from build123d import *

# Parameters (mm, degrees)
TD_SKETCH_R                             = 0.79248
TL_FEATURE_DEPTH                        = 21.0312
TDF_STD_SKETCH_W                        = 2.09296
TDF_STD_SKETCH_H                        = 2.09296
TDF_STD_FEATURE_DEPTH                   = 22.061040395
ISA_20_STD_FEATURE_DEPTH                = 22.061040395
ISA_20_STD_FEATURE_DEPTH_BACK           = 22.061040395
F_10BA_STD_FEATURE_DEPTH                = 22.061040395
F_10BA_STD_FEATURE_DEPTH_BACK           = 22.061040395
FRO_STD_FEATURE_DEPTH                   = 22.061040395
FRO_STD_FEATURE_DEPTH_BACK              = 22.061040395
C_STD_FEATURE_DEPTH                     = 22.061040395
C_STD_FEATURE_DEPTH_BACK                = 22.061040395
ERW_STD_FEATURE_DEPTH                   = 0.0254
H_STD_FEATURE_REACH                     = 22.907
H_STD_SKETCH_R                          = 0.0254
H_STD_SKETCH_3_R                        = 0.0254
FUNNEL_FINAL_DIAMETRE_STD_FEATURE_DEPTH = 2.499995
FUNNEL_FINAL_DIAMETRE_STD_FEATURE_DRAFT = -22.5
ROUND_BR_STD_FEATURE_START              = -1
ROUND_BR_STD_FEATURE_DEPTH              = 0.984425518


with BuildPart() as part:
    # TD_sketch → TL_feature (new body)
    with BuildSketch(Plane(origin=(0, 0, 0), x_dir=(1, 0, 0), z_dir=(0, 1, 0))):
        with Locations(Location((0, 0, 0), (0, 0, 270))):
            Circle(TD_SKETCH_R)
    extrude(amount=TL_FEATURE_DEPTH)

    # TDF_STD_sketch → TDF_STD_feature (cut, through all)
    with BuildSketch(Plane(origin=(0, 0, 0), x_dir=(1, 0, 0), z_dir=(0, 1, 0))):
        with Locations((-1.4224, 0)):
            Rectangle(TDF_STD_SKETCH_W, TDF_STD_SKETCH_H)
    extrude(amount=TDF_STD_FEATURE_DEPTH, mode=Mode.SUBTRACT)

    # ISA_20_STD_sketch → ISA_20_STD_feature (cut, two sides: drawn at the far end of the back side and taken through both)
    with BuildSketch(Plane(origin=(0, 0, 0), x_dir=(0, 0, -1), z_dir=(1, 0, 0)).offset(-ISA_20_STD_FEATURE_DEPTH_BACK)):
        Polygon((-12.968809457, 73.261672178), (-3.759167997, 21.0312), (-0.0508, 0), (0.0508, 0), (3.759167997, 21.0312), (12.968809457, 73.261672178), (12.968809457, -32.810750623), (-12.968809457, -32.810750623), align=None)
    extrude(amount=ISA_20_STD_FEATURE_DEPTH + ISA_20_STD_FEATURE_DEPTH_BACK, mode=Mode.SUBTRACT)

    # 10BA_STD_sketch → 10BA_STD_feature (cut, two sides: drawn at the far end of the back side and taken through both)
    with BuildSketch(Plane.XY.offset(-F_10BA_STD_FEATURE_DEPTH_BACK)):
        Polygon((-53.226091717, 0), (-0.37592, 0), (-0.24892, 0), (0.011534356, 0.036604473), (3.713447997, 21.0312), (12.890784005, 73.078458855), (91.272293615, 2.163710365), (25.155417893, -70.914748491), align=None)
    extrude(amount=F_10BA_STD_FEATURE_DEPTH + F_10BA_STD_FEATURE_DEPTH_BACK, mode=Mode.SUBTRACT)

    # FRO_STD_sketch → FRO_STD_feature (cut, two sides: drawn at the far end of the back side and taken through both)
    with BuildSketch(Plane.XY.offset(-FRO_STD_FEATURE_DEPTH_BACK)):
        with BuildLine():
            Line((-0.37592, 52.149873762), (-0.37592, 0.0254))
            ThreePointArc((-0.37592, 0.0254), (-0.368480512, 0.007439488), (-0.35052, 0))
            Line((-0.35052, 0), (51.773953762, 0))
            Line((51.773953762, 0), (-21.941183964, -73.715137726))
            Line((-21.941183964, -73.715137726), (-74.091057726, -21.565263964))
            Line((-74.091057726, -21.565263964), (-0.37592, 52.149873762))
        make_face()
    extrude(amount=FRO_STD_FEATURE_DEPTH + FRO_STD_FEATURE_DEPTH_BACK, mode=Mode.SUBTRACT)

    # C_STD_sketch → C_STD_feature (cut, two sides: drawn at the far end of the back side and taken through both)
    with BuildSketch(Plane(origin=(0, 0, 0), x_dir=(0, 0, -1), z_dir=(1, 0, 0)).offset(-C_STD_FEATURE_DEPTH_BACK)):
        with BuildLine():
            Line((-51.498419713, -8.177529753), (-0.048243287, 0))
            ThreePointArc((-0.048243287, 0), (0, 0.00381), (0.048243287, 0))
            Line((0.048243287, 0), (51.498419713, -8.177529753))
            Line((51.498419713, -8.177529753), (51.498419713, -112.369518834))
            Line((51.498419713, -112.369518834), (-51.498419713, -112.369518834))
            Line((-51.498419713, -112.369518834), (-51.498419713, -8.177529753))
        make_face()
    extrude(amount=C_STD_FEATURE_DEPTH + C_STD_FEATURE_DEPTH_BACK, mode=Mode.SUBTRACT)


with BuildPart() as body_2:
    # ERW_STD_sketch → ERW_STD_feature (new, symmetric)
    with BuildSketch(Plane.XY):
        Polygon((-0.127, 0.0762), (-0.127, 0), (-0.29718, 0), (-0.239759181, 0.0762), align=None)
    extrude(amount=ERW_STD_FEATURE_DEPTH, both=True)

    # H_STD_sketch → H_STD_feature (add, up to next)
    with BuildSketch(Plane(origin=(0.008335492, 0.154335983, 0), x_dir=(0, 0, -1), z_dir=(0.8660254037844415, 0.4999999999999953, 0)), mode=Mode.PRIVATE) as h_std_feature_sk1:
        with Locations(Location((0, 0, 0), (0, 0, 90))):
            Circle(H_STD_SKETCH_R)
    h_std_feature_tool1 = extrude(h_std_feature_sk1.sketch, amount=-H_STD_FEATURE_REACH, mode=Mode.PRIVATE) - body_2.part
    add(h_std_feature_tool1.solids().sort_by_distance((0.008335, 0.154336, 0))[0])


with BuildPart() as funnel_final_diametre_std_feature_tool:
    # H_STD_sketch<3> → funnel_final_diametre_STD_feature (with draft: the straight prism first)
    with BuildSketch(Plane(origin=(0.008335492, 0.154335983, 0), x_dir=(0, 0, -1), z_dir=(0.8660254037844415, 0.4999999999999953, 0))):
        with Locations(Location((0, 0, 0), (0, 0, 90))):
            Circle(H_STD_SKETCH_3_R)
    extrude(amount=FUNNEL_FINAL_DIAMETRE_STD_FEATURE_DEPTH)
    # funnel_final_diametre_STD_feature: the draft: its side faces are tilted about the plane it starts from
    funnel_final_diametre_std_feature_sides = [funnel_final_diametre_std_feature_tool.faces().sort_by_distance(p)[0] for p in [
        (1.103565082, 0.757337687, 0),
    ]]
    draft(funnel_final_diametre_std_feature_sides, Plane(origin=(0.008335492, 0.154335983, 0), x_dir=(0, 0, -1), z_dir=(0.8660254037844415, 0.4999999999999953, 0)), FUNNEL_FINAL_DIAMETRE_STD_FEATURE_DRAFT)


with BuildPart() as body_2_1:
    add(body_2.part)

    # funnel_final_diametre_STD_feature: add funnel_final_diametre_std_feature_tool
    add(funnel_final_diametre_std_feature_tool.part)

    # ROUND_BR_STD_feature: read off the stored shape, not the designer's step
    # ROUND_BR_STD_feature outline → ROUND_BR_STD_feature (cut)
    with BuildSketch(Plane(origin=(0, 0, 0), x_dir=(0.79863551004729, -0.601815023152052, 0), z_dir=(0.601815023152052, 0.79863551004729, 0)).offset(ROUND_BR_STD_FEATURE_START)):
        with BuildLine():
            Line((-0.237338501, -0.0254), (-0.211938501, -0.0254))
            ThreePointArc((-0.211938501, -0.0254), (-0.229899013, -0.017960512), (-0.237338501, 0))
            Line((-0.237338501, 0), (-0.237338501, -0.0254))
        make_face()
        with BuildLine():
            Line((-0.237338501, 0.0254), (-0.237338501, 0))
            ThreePointArc((-0.237338501, 0), (-0.229899013, 0.017960512), (-0.211938501, 0.0254))
            Line((-0.211938501, 0.0254), (-0.237338501, 0.0254))
        make_face()
    extrude(amount=ROUND_BR_STD_FEATURE_DEPTH, mode=Mode.SUBTRACT)


with BuildPart() as part_1:
    add(part.part)

    # COMBINE_STD_feature: cut body 2
    add(body_2_1.part, mode=Mode.SUBTRACT)


solid = part_1.part
Here's how the part is built. I have some questions about the finished solid (model axes, mm). Coordinates: 2 decimals unless noted, no trailing zeros. Loops run counter-clockwise (first coordinate to the right, second up) from the corner with the lowest first, then second, coordinate; pieces in that order, holes last. Notation, with made-up numbers: (-5.5, -1) -> (37.5, -1) arc R30 ccw to (37.5, 22) -> close; hole circle Ø6 at (34, 1.5). An arc over 180 degrees is marked (long way). Use one line per item in the form item = value. Start each with the question number.
(1) If we section it at C-C (y = 1.75): Please give me the cut outline in (x, z).
(2) If we section it at B-B (z = 0.3): Please give me the cut outline in (x, y), then the cut area to 3 significant figures.
(3) Please list where these lines run through material, in increasing order: line 1 along Z through (x, y) = (-0.05, 18); line 2 along X through (y, z) = (2, -0.35); line 3 along Z through (x, y) = (0.65, 13.5).
(4) If we section it at A-A (y = 7): Please give me the cut outline in (x, z), then the cut area to 3 significant figures.
Verdict:
q1.outline = (-0.38, -0.36) -> (0.31, -0.36) -> (0.31, 0.36) -> (-0.38, 0.36) -> close
q2.outline = (-0.38, 1.41) -> (0.25, 1.41) -> (0.73, 4.13) -> (0.73, 21.03) -> (-0.38, 21.03) -> close
q2.area = 21.1 mm²
q3.line_1 = -0.79 to 0.79
q3.line_2 = -0.38 to 0.36
q3.line_3 = -0.45 to 0.45
q4.outline = (-0.38, -0.7) arc R0.79 ccw (long way) to (-0.38, 0.7) -> close
q4.area = 1.56 mm²
